Source: CAD feature listing. Evaluate the final solid. Frame: model axes, mm. A direction names the side the tool comes from. Give positions to 0.01 mm unless a question says otherwise; leave off trailing zeros. Write each loop counter-clockwise with the first axis right and the second up, starting at its lowest first coordinate (ties: lowest second). Pieces come first, ordered by that corner, then holes. Notation, with made-up numbers: (-18.5, 58) -> (-8.5, 58) arc R13 ccw to (-8.5, 81) -> close; hole circle Ø5 at (33, 25.5). An arc over 180 degrees is marked (long way). Answer as a JSON object with one key per item and string values. Group by question number.
Item 1: Section query B-B on x = -9. Return the cut outline in (y, z).
Item 2: Pull-direction query (Z, two-part tool) for faces 6 (the face through (25.4, 50, 2)), 7 (the face through (22.86, 26, 0)), 8 (the face through (-2, 50, 25.4)); classes: pulls with the +Z half, pulls with the -Z half, needs draft (parallel to the pull), parting line crosses it, or undercut.
Item 3: Section query A-A on y = 8. Return the cut outline in (x, z), plus the area to 3 significant figures.
Item 4: First-contact query: pin 1 Ø23 at (x, y) = (7.5, 26) entering from +Z; pin 2 Ø5 at (x, y) = (-13.5, 28) entering from -Z; pin 3 Ø3 at (y, z) = (9.5, -14) entering from +X; pin 4 Ø1.4 at (x, z) = (24.5, -1) entering from -Y. Flat tips, straight axial feed; report the tip coordinate or a pass-through.
Item 5: Section query C-C on z = -18. Return the cut outline in (x, y), plus the area to 3 significant figures.
Item 6: Access query for faces 1 (the face through (0, 2.54, 0)), 2 (the face through (-24.13, 26, 0)), 3 (the face through (0, 26, -24.13)), 4 (the face through (24.13, 26, 0)), 5 (the face through (0, 26, 24.13)). Directions: +Z, -Z, +X, -X, +Y, -Y. A direction counts if a zero-diameter tool reaches every point of the face in a straight line with its end or side. Return the directions, or none.
Item 7: Ray query, probe 1 along Z at (x, y) = (-10, 33.5); probe 2 along Y at (x, z) = (-2.5, -10). Return the intervals inside material, ascending. Write a range as from..to.
from build123d import *

# Parameters (mm, degrees)
SKETCH1_W           = 50.8
SKETCH1_H           = 50.8
BOSS_EXTRUDE1_DEPTH = 50.8
SHELL1_T            = -2.54
SKETCH2_W           = 45.72
SKETCH2_H           = 45.72
CUT_EXTRUDE1_DEPTH  = 1.27
SKETCH3_W           = 45.72
SKETCH3_H           = 45.72
CUT_EXTRUDE2_DEPTH  = 1.27
SKETCH4_W           = 45.72
SKETCH4_H           = 45.72
CUT_EXTRUDE3_DEPTH  = 1.27
SKETCH5_W           = 45.72
SKETCH5_H           = 45.72
CUT_EXTRUDE4_DEPTH  = 1.27


with BuildPart() as part:
    # Sketch1 → Boss-Extrude1 (new body)
    with BuildSketch(Plane(origin=(0, 0, 0), x_dir=(1, 0, 0), z_dir=(0, 1, 0))):
        Rectangle(SKETCH1_W, SKETCH1_H)
    extrude(amount=BOSS_EXTRUDE1_DEPTH)

    # Shell1
    shell1_openings = [part.faces().sort_by_distance(p)[0] for p in [
        (0, 50.8, 0),
    ]]
    offset(amount=SHELL1_T, openings=shell1_openings, kind=Kind.INTERSECTION)

    # Sketch2 → Cut-Extrude1 (cut)
    with BuildSketch(Plane.XY.offset(25.4)):
        with Locations((0, 25.4)):
            Rectangle(SKETCH2_W, SKETCH2_H)
    extrude(amount=-CUT_EXTRUDE1_DEPTH, mode=Mode.SUBTRACT)

    # Sketch3 → Cut-Extrude2 (cut)
    with BuildSketch(Plane(origin=(25.4, 0, 0), x_dir=(0, 0, -1), z_dir=(1, 0, 0))):
        with Locations((0, 25.4)):
            Rectangle(SKETCH3_W, SKETCH3_H)
    extrude(amount=-CUT_EXTRUDE2_DEPTH, mode=Mode.SUBTRACT)

    # Sketch4 → Cut-Extrude3 (cut)
    with BuildSketch(Plane(origin=(0, 0, -25.4), x_dir=(-1, 0, 0), z_dir=(0, 0, -1))):
        with Locations((0, 25.4)):
            Rectangle(SKETCH4_W, SKETCH4_H)
    extrude(amount=-CUT_EXTRUDE3_DEPTH, mode=Mode.SUBTRACT)

    # Sketch5 → Cut-Extrude4 (cut)
    with BuildSketch(Plane.ZY.offset(25.4)):
        with Locations((0, 25.4)):
            Rectangle(SKETCH5_W, SKETCH5_H)
    extrude(amount=-CUT_EXTRUDE4_DEPTH, mode=Mode.SUBTRACT)


solid = part.part
Worked answers:
{
 "1": {"outline": "(0, -25.4) -> (2.54, -25.4) -> (2.54, -24.13) -> (48.26, -24.13) -> (48.26, -25.4) -> (50.8, -25.4) -> (50.8, -22.86) -> (2.54, -22.86) -> (2.54, 22.86) -> (50.8, 22.86) -> (50.8, 25.4) -> (48.26, 25.4) -> (48.26, 24.13) -> (2.54, 24.13) -> (2.54, 25.4) -> (0, 25.4) -> close"},
 "2": {"face 6": "needs draft", "face 7": "undercut", "face 8": "pulls with the +Z half"},
 "3": {"outline": "(-25.4, -25.4) -> (-22.86, -25.4) -> (-22.86, -24.13) -> (22.86, -24.13) -> (22.86, -25.4) -> (25.4, -25.4) -> (25.4, -22.86) -> (24.13, -22.86) -> (24.13, 22.86) -> (25.4, 22.86) -> (25.4, 25.4) -> (22.86, 25.4) -> (22.86, 24.13) -> (-22.86, 24.13) -> (-22.86, 25.4) -> (-25.4, 25.4) -> (-25.4, 22.86) -> (-24.13, 22.86) -> (-24.13, -22.86) -> (-25.4, -22.86) -> close; hole (-22.86, -22.86) -> (22.86, -22.86) -> (22.86, 22.86) -> (-22.86, 22.86) -> close", "area": "258 mm^2"},
 "4": {"pin 1": "z = 24.13", "pin 2": "z = -24.13", "pin 3": "x = 24.13", "pin 4": "y = 0"},
 "5": {"outline": "(-25.4, 0) -> (25.4, 0) -> (25.4, 2.54) -> (24.13, 2.54) -> (24.13, 48.26) -> (25.4, 48.26) -> (25.4, 50.8) -> (22.86, 50.8) -> (22.86, 2.54) -> (-22.86, 2.54) -> (-22.86, 50.8) -> (-25.4, 50.8) -> (-25.4, 48.26) -> (-24.13, 48.26) -> (-24.13, 2.54) -> (-25.4, 2.54) -> close", "area": "258 mm^2"},
 "6": {"face 1": "+Y", "face 2": "-X", "face 3": "-Z", "face 4": "+X", "face 5": "+Z"},
 "7": {"probe 1": "-24.13..-22.86, 22.86..24.13", "probe 2": "0..2.54"}
}
